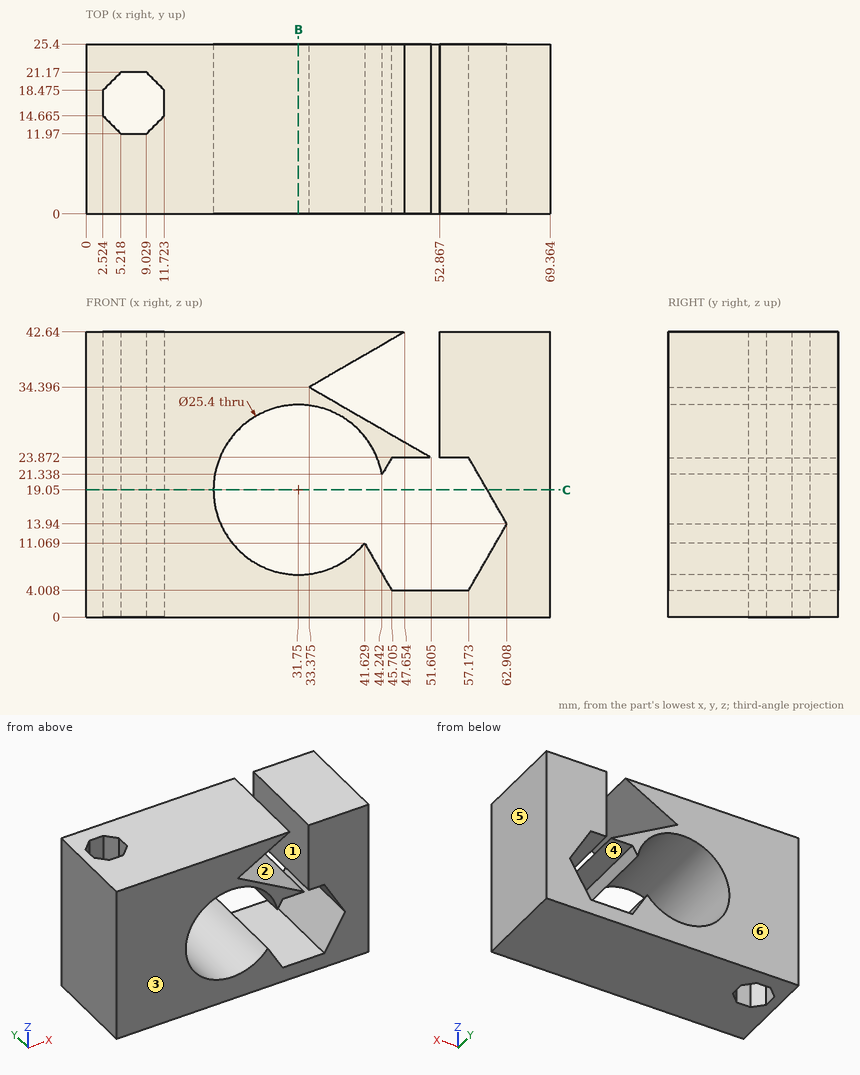
Part print with two shaded views. Sizes in mm from the minimum x, y, z corner. A direction names the side the tool comes from. Round coordinates to 2 decimals unless told otherwise and drop trailing zeros. Order: outer loops, then holes, each group sorted by start corner. A loop starts at its lowest first (then second) coordinate and runs counter-clockwise, first axis right, second up.
(1) Drill centre lines: line 1 (Z direction, x = 31.75, y = 9.25); line 2 (X direction, y = 15, z = 10.5) (1 decimal); line 3 (Z direction, x = 58, y = 18). Where is each one in solid material? Low to high.
(2) Pull direction X, two halves, no side cores. Call the marked faces 4, 5 and 6: released by +X, released by -X, zero draft, split by the parting line, or undercut.
(3) 3-axis set-ups, long thin cutter, end or side, ignore diameter. For the marked faces 1, 2 and 3: which of +Z, -Z, +X, -X, +Y, -Y reach the whole face in a straight line?
(4) Band-saw the part on C-C (z = 19.05). Give the number of separate pieces and of enclosed holes in the cut face, then the cut area to 3 significant figures.
(5) Band-saw the part on B-B (x = 31.75). List the corners of the cut face in (y, z).
(6) Pin check, flat tip, straight feed: pin 1 (6 mm diameter, centred on x = 23, z = 16, fed in from -Y). Stop position of the tip, or through.
Verdict:
1. line 1: z = 0 to 6.35, 31.75 to 42.64
1. line 2: x = 0 to 2.5, 11.7 to 22.4, 41.1 to 42, 60.9 to 69.4
1. line 3: z = 0 to 5.44, 22.44 to 42.64
2. face 4: undercut
2. face 5: released by +X
2. face 6: zero draft
3. face 1: +Z, +Y, -Y
3. face 2: +Y, -Y
3. face 3: +Z, -Z, +X, -X, -Y
4. separate pieces: 2
4. enclosed holes: 1
4. area: 653 mm2
5. outline: (0, 0) - (25.4, 0) - (25.4, 6.35) - (0, 6.35) - close; (0, 31.75) - (25.4, 31.75) - (25.4, 42.64) - (0, 42.64) - close
6. pin 1: passes through
